```python
from build123d import *

# Parameters (mm, degrees)
SKETCH1_R                        = 15
BOSS_EXTRUDE1_DEPTH              = 195.5
SKETCH2_OUTSIDE_W                = 110.66
SKETCH2_OUTSIDE_H                = 110.66
SKETCH2_OUTSIDE_R                = 12
CUT_EXTRUDE1_DEPTH               = 10
F_13_5_13_5_DIAMETER_HOLE1_D     = 13.5
F_13_5_13_5_DIAMETER_HOLE1_DEPTH = 2
F_13_5_13_5_DIAMETER_HOLE1_TIP   = 4.055809178


with BuildPart() as part:
    # Sketch1 → Boss-Extrude1 (new, symmetric)
    with BuildSketch(Plane(origin=(0, 0, 0), x_dir=(1, 0, 0), z_dir=(0, 1, 0))):
        with Locations(Location((0, 0, 0), (0, 0, 270))):
            Circle(SKETCH1_R)
    extrude(amount=BOSS_EXTRUDE1_DEPTH, both=True)

    # Sketch2 outside → Cut-Extrude1 (cut)
    with BuildSketch(Plane(origin=(0, 195.5, 0), x_dir=(1, 0, 0), z_dir=(0, 1, 0))):
        Rectangle(SKETCH2_OUTSIDE_W, SKETCH2_OUTSIDE_H)
        with Locations(Location((0, 0, 0), (0, 0, 270))):
            Circle(SKETCH2_OUTSIDE_R, mode=Mode.SUBTRACT)
    cut_extrude1 = extrude(amount=-CUT_EXTRUDE1_DEPTH, mode=Mode.SUBTRACT)

    # Mirror1: Cut-Extrude1 across plane
    add(cut_extrude1.mirror(Plane.ZX), mode=Mode.SUBTRACT)

    # Ø13.5 (13.5) Diameter Hole1
    with Locations(Plane(origin=(0, -195.5, 0), x_dir=(-1, 0, 0), z_dir=(0, -1, 0))):
        with Locations((0, 0)):
            Hole(F_13_5_13_5_DIAMETER_HOLE1_D / 2, depth=F_13_5_13_5_DIAMETER_HOLE1_DEPTH)
            with Locations((0, 0, -(F_13_5_13_5_DIAMETER_HOLE1_DEPTH + F_13_5_13_5_DIAMETER_HOLE1_TIP / 2))):  # 118° drill point
                Cone(0, F_13_5_13_5_DIAMETER_HOLE1_D / 2, F_13_5_13_5_DIAMETER_HOLE1_TIP, mode=Mode.SUBTRACT)


solid = part.part
```
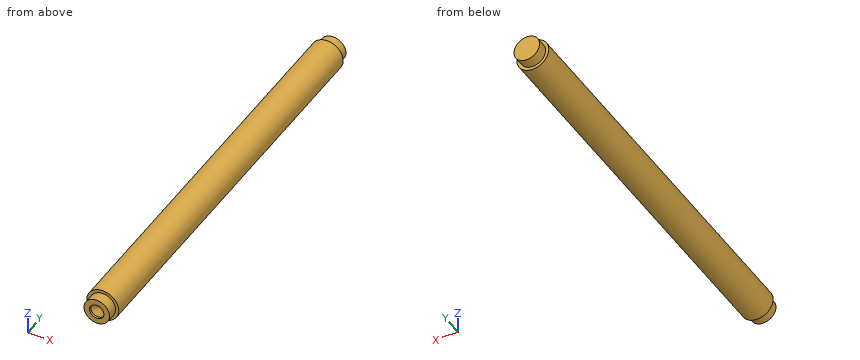
Geometry check sheet. Reference: the model listing, model coordinates, mm. Coordinates: 2 decimals unless noted, no trailing zeros. Loops run counter-clockwise (first coordinate to the right, second up) from the corner with the lowest first, then second, coordinate; pieces in that order, holes last. Notation, with made-up numbers: (-12, 36.25) -> (3, 36.25) arc R31 ccw to (3, 75.25) -> close; hole circle Ø4 at (-15, 23). An arc over 180 degrees is marked (long way). Put each result on its own line as item: value.
1) Cross-section at A-A on y = 106. Record the boundary of the cut face in (x, z).
Result set:
outline: circle Ø30 at (0, 0)
2) Gauge pin test, flat ends, axial feed: pin 1 Ø1.5 at (x, y) = (8.5, 83) entering from -Z; pin 2 Ø10 at (y, z) = (109, -11) entering from +X; pin 3 Ø10 at (x, y) = (-11.5, 81.5) entering from -Z. Record the tip position at first contact, or that the pin passes through.
Result set:
pin 1: stops at z = -12.84
pin 2: stops at x = 13.75
pin 3: stops at z = -13.52
3) Thickness scan on line 1 (Y direction, x = 11.5, z = -7); line 2 (Z direction, x = 9, y = 75.5); line 3 (X direction, y = 117, z = -1.25). Record the ranges inside material, lowest first.
Result set:
line 1: y = -185.5 to 185.5
line 2: z = -12 to 12
line 3: x = -14.95 to 14.95
